Part print with two shaded views. Sizes in mm from the minimum x, y, z corner. Round coordinates to 2 decimals unless told otherwise and drop trailing zeros. Write each loop counter-clockwise with the first axis right and the second up, starting at its lowest first coordinate (ties: lowest second). Pieces come first, ordered by that corner, then holes. Notation, with made-up numbers: (40, -39.5) - (77, -39.5) arc R20 ccw to (77, -16.5) - close; hole circle Ø1 at (40.25, 68.5). An arc over 180 degrees is marked (long way). Use one line per item in the form item = value. Start each with the question number.
Item 1: Pin check, flat tip, straight feed: pin 1 (8 mm diameter, centred on x = 25.5, z = 5, fed in from +Y). Stop position of the tip, or through.
Item 2: Band-saw the part on A-A, the plane z = 23. List the corners of the cut face in (x, y) (3 decimals).
Item 3: Drill centre lines: L1, parallel to Z at x = 12.5, y = 0.2 (3 decimals); L2, parallel to X at y = 1.2, z = 34.5 (3 decimals); L3, parallel to X at y = 1.5, z = 46. Where is each one in solid material? Low to high.
Item 4: Band-saw the part on B-B, the plane x = 48. List the corners of the cut face in (y, z) (3 decimals), and give its area (3 significant figures).
Item 5: Band-saw the part on C-C, the plane y = 0.55. Give the number of separate pieces and of enclosed holes in the cut face, and give its area (3 significant figures).
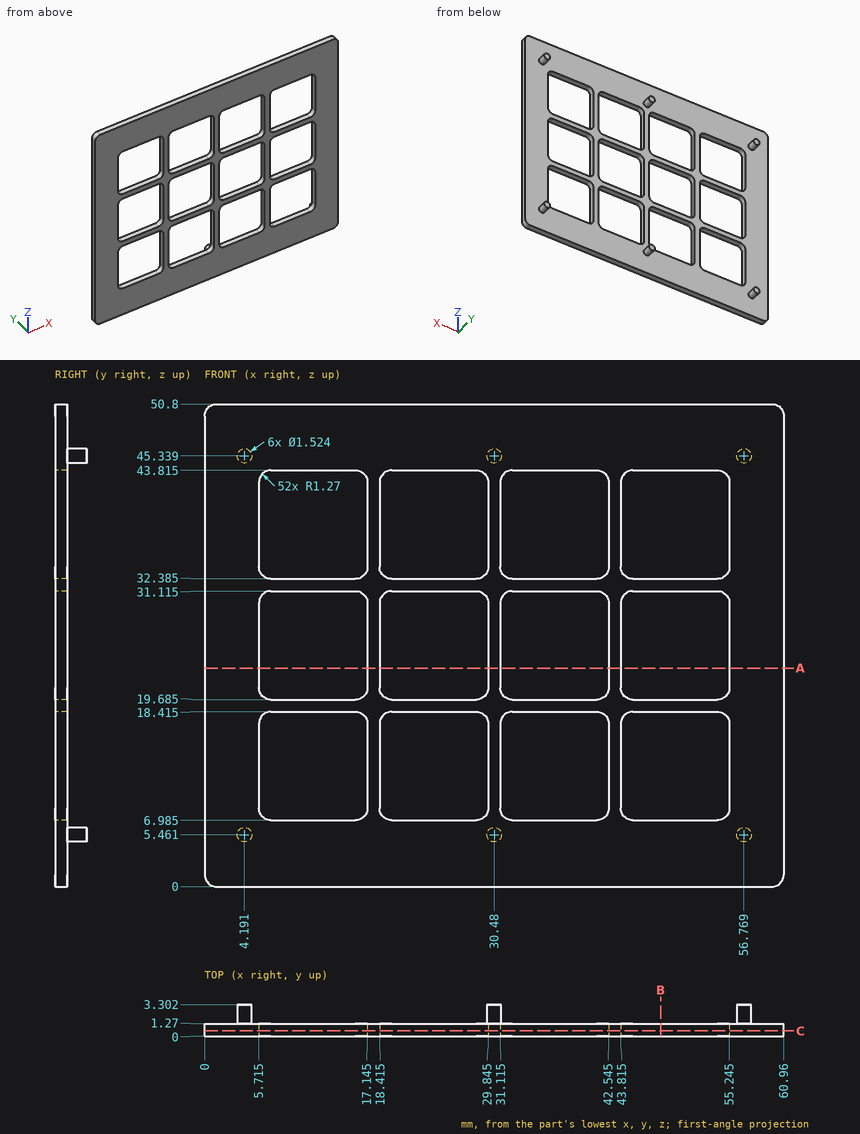
Determined:
q1.pin_1 = 1.27
q2.outline = (0, 0) - (5.715, 0) - (5.715, 1.27) - (0, 1.27) - close; (17.145, 0) - (18.415, 0) - (18.415, 1.27) - (17.145, 1.27) - close; (29.845, 0) - (31.115, 0) - (31.115, 1.27) - (29.845, 1.27) - close; (42.545, 0) - (43.815, 0) - (43.815, 1.27) - (42.545, 1.27) - close; (55.245, 0) - (60.96, 0) - (60.96, 1.27) - (55.245, 1.27) - close
q3.L1 = 0 to 6.985, 18.415 to 19.685, 31.115 to 32.385, 43.815 to 50.8
q3.L2 = 0 to 5.715, 17.145 to 18.415, 29.845 to 31.115, 42.545 to 43.815, 55.245 to 60.96
q3.L3 = 3.81 to 4.57, 30.1 to 30.86, 56.39 to 57.15
q4.outline = (0, 0) - (1.27, 0) - (1.27, 6.985) - (0, 6.985) - close; (0, 18.415) - (1.27, 18.415) - (1.27, 19.685) - (0, 19.685) - close; (0, 31.115) - (1.27, 31.115) - (1.27, 32.385) - (0, 32.385) - close; (0, 43.815) - (1.27, 43.815) - (1.27, 50.8) - (0, 50.8) - close
q4.area = 21.0 mm²
q5.separate_pieces = 1
q5.enclosed_holes = 12
q5.area = 1,540 mm²
